Can you work these out from the model? Positions are in its coordinate system, mm. Give positions to 0.01 mm unless a question says otherwise; leave off trailing zeros. Write each loop counter-clockwise with the first axis right and the second up, starting at its lowest first coordinate (ties: lowest second). Pieces come first, ordered by that corner, then holes. Notation, with made-up numbers: M 62,13 L 83,13 A20 ccw 83,38 Z; hole C 16,-22.75 d10. An arc over 180 degrees is marked long. Write each question's results on one line, items separated by ' | '.
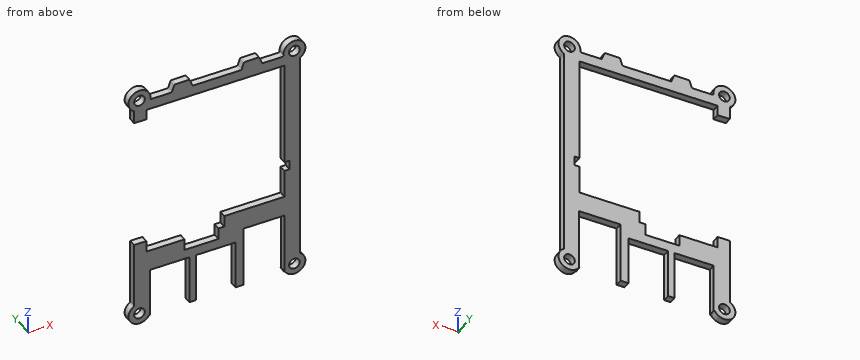
from build123d import *

# Parameters (mm, degrees)
BASEPLATE_OUTLINE_R = 2.1
BASEPLATE_DEPTH     = 2.8
CUT_EXTRUDE1_REACH  = 115.438
SKETCH3_W           = 15.4
SKETCH3_H           = 19.2
SKETCH3_W_2         = 15.6
SKETCH3_W_3         = 16.2
SKETCH3_H_2         = 24


# Read off the part's stored shape, not the designer's step: BasePlate
with BuildPart() as part:
    # BasePlate outline → BasePlate (new body)
    with BuildSketch(Plane(origin=(0, 0, 0), x_dir=(1, 0, 0), z_dir=(0, 1, 0))):
        with BuildLine():
            Line((43.502626614, -5.852332608), (48.792614178, -5.852332608))
            ThreePointArc((48.792614178, -5.852332608), (49.082078508, -5.760021707), (49.264659986, -5.517174213))
            Line((49.264659986, -5.517174213), (50.078201202, -3.187491002))
            ThreePointArc((50.078201202, -3.187491002), (50.26078268, -2.944643509), (50.55024701, -2.852332608))
            Line((50.55024701, -2.852332608), (58.116695703, -2.852332608))
            ThreePointArc((58.116695703, -2.852332608), (58.484685739, -3.013831008), (58.614956567, -3.393999275))
            ThreePointArc((58.614956567, -3.393999275), (64.799237397, -7.61016844), (65.229166667, -0.137781095))
            ThreePointArc((65.229166667, -0.137781095), (65.061014427, 0.043158816), (65, 0.282515593))
            Line((65, 0.282515593), (65, 83.012819192))
            ThreePointArc((65, 83.012819192), (65.061014427, 83.252175969), (65.229166667, 83.433115879))
            ThreePointArc((65.229166667, 83.433115879), (65.940559159, 90.088226551), (59.285448487, 89.376834059))
            ThreePointArc((59.285448487, 89.376834059), (59.104508577, 89.208681819), (58.8651518, 89.147667392))
            Line((58.8651518, 89.147667392), (6.1348482, 89.147667392))
            ThreePointArc((6.1348482, 89.147667392), (5.895491423, 89.208681819), (5.714551513, 89.376834059))
            ThreePointArc((5.714551513, 89.376834059), (-0.940559159, 90.088226551), (-0.229166667, 83.433115879))
            ThreePointArc((-0.229166667, 83.433115879), (-0.061014427, 83.252175969), (0, 83.012819192))
            Line((0, 83.012819192), (0, 0.282515593))
            ThreePointArc((0, 0.282515593), (-0.061014427, 0.043158816), (-0.229166667, -0.137781095))
            ThreePointArc((-0.229166667, -0.137781095), (0.200762603, -7.61016844), (6.385043433, -3.393999275))
            ThreePointArc((6.385043433, -3.393999275), (6.515314261, -3.013831008), (6.883304297, -2.852332608))
            Line((6.883304297, -2.852332608), (14.44975299, -2.852332608))
            ThreePointArc((14.44975299, -2.852332608), (14.73921732, -2.944643509), (14.921798798, -3.187491002))
            Line((14.921798798, -3.187491002), (15.735340014, -5.517174213))
            ThreePointArc((15.735340014, -5.517174213), (15.917921492, -5.760021707), (16.207385822, -5.852332608))
            Line((16.207385822, -5.852332608), (21.497373386, -5.852332608))
            ThreePointArc((21.497373386, -5.852332608), (21.786837716, -5.760021707), (21.969419194, -5.517174213))
            Line((21.969419194, -5.517174213), (22.78296041, -3.187491002))
            ThreePointArc((22.78296041, -3.187491002), (22.965541888, -2.944643509), (23.255006218, -2.852332608))
            Line((23.255006218, -2.852332608), (41.744993782, -2.852332608))
            ThreePointArc((41.744993782, -2.852332608), (42.034458112, -2.944643509), (42.21703959, -3.187491002))
            Line((42.21703959, -3.187491002), (43.030580806, -5.517174213))
            ThreePointArc((43.030580806, -5.517174213), (43.213162284, -5.760021707), (43.502626614, -5.852332608))
        make_face()
        with Locations((2.1, -3.752332608)):
            Circle(BASEPLATE_OUTLINE_R, mode=Mode.SUBTRACT)
        with Locations((62.9, -3.752332608)):
            Circle(BASEPLATE_OUTLINE_R, mode=Mode.SUBTRACT)
        with Locations((2.1, 87.047667392)):
            Circle(BASEPLATE_OUTLINE_R, mode=Mode.SUBTRACT)
        with Locations((62.9, 87.047667392)):
            Circle(BASEPLATE_OUTLINE_R, mode=Mode.SUBTRACT)
    extrude(amount=BASEPLATE_DEPTH)

    # Sketch3 → Cut-Extrude1 (cut, up to next)
    with BuildSketch(Plane(origin=(0, 2.8, 0), x_dir=(1, 0, 0), z_dir=(0, 1, 0)), mode=Mode.PRIVATE) as cut_extrude1_sk1:
        Polygon((4.8, 1.147667392), (59, 1.147667392), (59, 42.447667392), (61, 42.447667392), (61, 46.147667392), (59, 46.147667392), (59, 57.147667392), (35.4, 57.147667392), (35.4, 61.647667392), (33.1, 61.647667392), (33.1, 66.147667392), (19.8, 66.147667392), (19.8, 61.647667392), (4.8, 61.647667392), (4.8, 57.147667392), (0, 57.147667392), (0, 5.147667392), (4.8, 5.147667392), align=None)
    cut_extrude1_tool1 = extrude(cut_extrude1_sk1.sketch, amount=-CUT_EXTRUDE1_REACH, mode=Mode.PRIVATE) & part.part
    # Sketch3 → Cut-Extrude1 (cut, up to next)
    with BuildSketch(Plane(origin=(0, 2.8, 0), x_dir=(1, 0, 0), z_dir=(0, 1, 0)), mode=Mode.PRIVATE) as cut_extrude1_sk2:
        with Locations((14, 79.547667392)):
            Rectangle(SKETCH3_W, SKETCH3_H)
    cut_extrude1_tool2 = extrude(cut_extrude1_sk2.sketch, amount=-CUT_EXTRUDE1_REACH, mode=Mode.PRIVATE) & part.part
    # Sketch3 → Cut-Extrude1 (cut, up to next)
    with BuildSketch(Plane(origin=(0, 2.8, 0), x_dir=(1, 0, 0), z_dir=(0, 1, 0)), mode=Mode.PRIVATE) as cut_extrude1_sk3:
        with Locations((32, 79.547667392)):
            Rectangle(SKETCH3_W_2, SKETCH3_H)
    cut_extrude1_tool3 = extrude(cut_extrude1_sk3.sketch, amount=-CUT_EXTRUDE1_REACH, mode=Mode.PRIVATE) & part.part
    # Sketch3 → Cut-Extrude1 (cut, up to next)
    with BuildSketch(Plane(origin=(0, 2.8, 0), x_dir=(1, 0, 0), z_dir=(0, 1, 0)), mode=Mode.PRIVATE) as cut_extrude1_sk4:
        with Locations((51, 77.147667392)):
            Rectangle(SKETCH3_W_3, SKETCH3_H_2)
    cut_extrude1_tool4 = extrude(cut_extrude1_sk4.sketch, amount=-CUT_EXTRUDE1_REACH, mode=Mode.PRIVATE) & part.part
    add(cut_extrude1_tool1.solids().sort_by_distance((29.290557, 2.8, -31.112428))[0], mode=Mode.SUBTRACT)
    add(cut_extrude1_tool2.solids().sort_by_distance((14, 2.8, -79.547667))[0], mode=Mode.SUBTRACT)
    add(cut_extrude1_tool3.solids().sort_by_distance((32, 2.8, -79.547667))[0], mode=Mode.SUBTRACT)
    add(cut_extrude1_tool4.solids().sort_by_distance((51, 2.8, -77.147667))[0], mode=Mode.SUBTRACT)


solid = part.part
Item 1: I want a section at A-A, the plane x = 62.9. Please give me the cut outline in (y, z).
Geometry says:
outline: M 0,-91.35 L 2.8,-91.35 L 2.8,-89.15 L 0,-89.15 Z; M 0,-84.95 L 2.8,-84.95 L 2.8,1.65 L 0,1.65 Z; M 0,5.85 L 2.8,5.85 L 2.8,8.05 L 0,8.05 Z
Item 2: I want a section at B-B, the plane x = 2.1. Please give me the cut outline in (y, z).
Geometry says:
outline: M 0,-91.35 L 2.8,-91.35 L 2.8,-89.15 L 0,-89.15 Z; M 0,-84.95 L 2.8,-84.95 L 2.8,-57.15 L 0,-57.15 Z; M 0,-5.15 L 2.8,-5.15 L 2.8,1.65 L 0,1.65 Z; M 0,5.85 L 2.8,5.85 L 2.8,8.05 L 0,8.05 Z
Item 3: If I drill on line 1 (Z direction, x = 62.9, y = 1.8); line 2 (Z direction, x = 2.1, y = 1.35); line 3 (X direction, y = 0.35, z = -79), over which ranges is the centre line in solid material (lowest first)? Write a range as from..to.
Geometry says:
line 1: z = -91.35..-89.15, -84.95..1.65, 5.85..8.05 | line 2: z = -91.35..-89.15, -84.95..-57.15, -5.15..1.65, 5.85..8.05 | line 3: x = 0..6.3, 21.7..24.2, 39.8..42.9, 59.1..65
Item 4: I want a section at D-D, the plane z = -37. Please give me the cut outline in (x, y).
Geometry says:
outline: M 59,0 L 65,0 L 65,2.8 L 59,2.8 Z
Item 5: I want a section at C-C, the plane x = 52.5. Please give me the cut outline in (y, z), and give its area (3 significant figures).
Geometry says:
outline: M 0,-65.15 L 2.8,-65.15 L 2.8,-57.15 L 0,-57.15 Z; M 0,-1.15 L 2.8,-1.15 L 2.8,2.85 L 0,2.85 Z | area: 33.6 mm2
Item 6: I'm going to push flat-ended pins straight in: pin 1 (0.8 mm diameter, centred on x = 23, y = 1.5, fed in from -Z); pin 2 (1.4 mm diameter, centred on y = 1, z = -81, fed in from +X); pin 3 (1 mm diameter, centred on x = 15, y = 2, fed in from -Z). Where does each tip first touch, or does it pass through?
Geometry says:
pin 1: stops at z = -89.15 | pin 2: stops at x = 65 | pin 3: stops at z = -69.95
